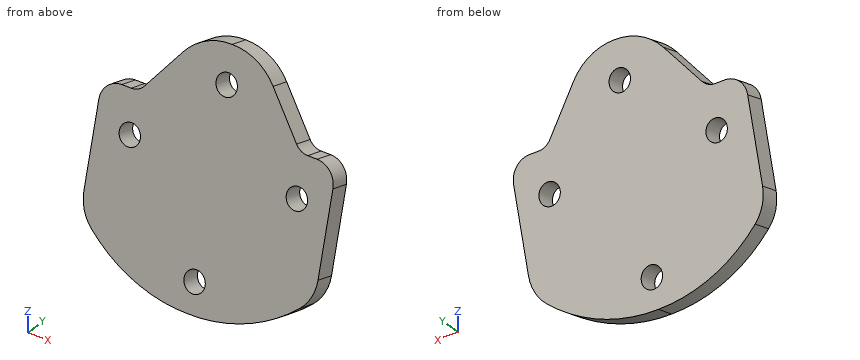
from build123d import *

# Parameters (mm, degrees)
SKETCH1_R      = 1.7272
EXTRUDE1_DEPTH = 3.175


with BuildPart() as part:
    # Sketch1 → Extrude1 (new body)
    with BuildSketch(Plane(origin=(0, 8.832630516, -2.366696214), x_dir=(1, 0, 0), z_dir=(0, 0.9659258262890681, -0.25881904510252135))):
        with BuildLine():
            Line((6.232958536, -16.463411329), (6.232958536, -29.501422299))
            ThreePointArc((6.232958536, -29.501422299), (5.303022566, -31.746486329), (3.057958536, -32.676422299))
            Line((3.057958536, -32.676422299), (1.503815544, -32.676422299))
            ThreePointArc((1.503815544, -32.676422299), (0.385985087, -32.93562089), (-0.503703576, -33.660315947))
            Line((-0.503703576, -33.660315947), (-5.578238388, -40.206928682))
            ThreePointArc((-5.578238388, -40.206928682), (-8.853459375, -42.848154666), (-12.965757523, -43.738183401))
            ThreePointArc((-12.965757523, -43.738183401), (-17.07805567, -42.848154665), (-20.353276656, -40.206928682))
            Line((-20.353276656, -40.206928682), (-25.427811468, -33.660315947))
            ThreePointArc((-25.427811468, -33.660315947), (-26.317500131, -32.93562089), (-27.435330589, -32.676422299))
            Line((-27.435330589, -32.676422299), (-28.98947358, -32.676422299))
            ThreePointArc((-28.98947358, -32.676422299), (-31.234537611, -31.746486329), (-32.16447358, -29.501422299))
            Line((-32.16447358, -29.501422299), (-32.16447358, -16.463411329))
            ThreePointArc((-32.16447358, -16.463411329), (-31.6135685, -13.876328394), (-30.056442678, -11.738139043))
            ThreePointArc((-30.056442678, -11.738139043), (-22.115977586, -6.903610393), (-12.965757522, -5.261317506))
            ThreePointArc((-12.965757522, -5.261317506), (-3.815537458, -6.903610394), (4.124927634, -11.738139043))
            ThreePointArc((4.124927634, -11.738139043), (5.682053455, -13.876328394), (6.232958536, -16.463411329))
        make_face()
        with Locations(Location((0.916706492, -26.332658417, 0), (0, 0, 270))):
            Circle(SKETCH1_R, mode=Mode.SUBTRACT)
        with Locations(Location((-12.782344336, -38.025699687, 0), (0, 0, 270))):
            Circle(SKETCH1_R, mode=Mode.SUBTRACT)
        with Locations(Location((-26.481395164, -26.332658417, 0), (0, 0, 270))):
            Circle(SKETCH1_R, mode=Mode.SUBTRACT)
        with Locations(Location((-12.782344336, -9.91136031, 0), (0, 0, 270))):
            Circle(SKETCH1_R, mode=Mode.SUBTRACT)
    extrude(amount=EXTRUDE1_DEPTH)


solid = part.part
Work out the finished part from the listing and answer in its coordinate system (mm). Give positions to 0.01 mm unless a question says otherwise; leave off trailing zeros. Write each loop counter-clockwise with the first axis right and the second up, starting at its lowest first coordinate (ties: lowest second). Pieces come first, ordered by that corner, then holes.
Q1. The part is cut by section A-A on x = -11.5. Give the vertices of the cut face in (y, z), and give its area (3 significant figures).
Answer:
outline: (10.2, 2.75) - (13.27, 1.92) - (14.17, 5.27) - (11.1, 6.09) - close; (11.7, 8.32) - (14.76, 7.5) - (21.44, 32.42) - (18.37, 33.25) - close; (18.97, 35.48) - (22.04, 34.66) - (23.2, 38.97) - (20.13, 39.79) - close
area: 107 mm2
Q2. The part is cut by section C-C on x = -5. Give the vertices of the cut face in (y, z).
Answer:
outline: (10.51, 3.9) - (13.58, 3.08) - (22.11, 34.93) - (19.05, 35.75) - close
Q3. The part is cut by section B-B on z = 15. Give the vertices of the cut face in (x, y), and give its area (3 significant figures).
Answer:
outline: (-32.16, 13.49) - (6.23, 13.49) - (6.23, 16.77) - (-32.16, 16.77) - close
area: 126 mm2
Q4. Given pin 1 (12 mm diameter, centred on x = 0.5, z = 22, fed in from -Y); pin 2 (1.5 mm diameter, centred on x = -13.5, z = 15, fed in from +Y); pin 3 (6 mm diameter, centred on y = 12.5, z = 20.5, fed in from +X), each flat-ended and moving along its own axis, determine where each tip first touches the part or whether it passes through.
Answer:
pin 1: stops at y = 13.75
pin 2: stops at y = 16.97
pin 3: stops at x = 6.23
Q5. Straight lines are drawn through the part: L1, parallel to Y at x = -27.5, z = 18.5; L2, parallel to Y at x = -21.5, z = 32.5; L3, parallel to X at y = 22.25, z = 37. For each, find the intervals that lie inside material, in ascending order.
Answer:
L1: y = 14.42 to 17.71
L2: y = 18.18 to 21.46
L3: x = -19.13 to -6.8
